Build history of the part. All positions in model axes, mm. A direction names the side the tool comes from. Coordinates: 2 decimals unless noted, no trailing zeros. Write each loop counter-clockwise with the first axis right and the second up, starting at its lowest first coordinate (ties: lowest second). Pieces come first, ordered by that corner, then holes.
```python
from build123d import *

# Parameters (mm, degrees)
SKETCH_1_R                  = 7.5
SKETCH_1_R_2                = 6
EXTRUDE_1_DEPTH             = 17
CUT_EXTRUDE_1_REACH         = 25.88
CUT_EXTRUDE_1_END_RADIUS    = 6
SKETCH_2_W                  = 1
SKETCH_2_H                  = 17
SKETCH_3_W                  = 4
SKETCH_3_H                  = 17
EXTRUDE_2_DEPTH             = 5
EXTRUDE_2_DIRECTION_2_REACH = 25.88
CUT_EXTRUDE_START           = -2
CUT_EXTRUDE_4_DEPTH         = 2
CUT_EXTRUDE_2_REACH         = 26.274
SKETCH_4_R                  = 1.25
CUT_EXTRUDE_3_DEPTH         = 1.5
EXTRUDE_6_DEPTH             = 5
SKETCH_13_W                 = 4.5
SKETCH_13_H                 = 12.5
EXTRUDE_7_DEPTH             = 5
CUT_EXTRUDE_5_REACH         = 34.2
SKETCH_11_R                 = 1.1
FILLET_1_R                  = 1.5


with BuildPart() as part:
    # 草图1 → 凸台-拉伸1 (new body)
    with BuildSketch(Plane(origin=(0, 0, 0), x_dir=(1, 0, 0), z_dir=(0, 1, 0))):
        with Locations(Location((0, 0, 0), (0, 0, 270))):
            Circle(SKETCH_1_R)
        with Locations(Location((0, 0, 0), (0, 0, 270))):
            Circle(SKETCH_1_R_2, mode=Mode.SUBTRACT)
    extrude(amount=EXTRUDE_1_DEPTH)

    # 切除-拉伸1: up to this cylinder (the profile starts outside it)
    cut_extrude_1_end = Plane(origin=(0, 8.5, 0), z_dir=(0, -1, 0)) * Cylinder(CUT_EXTRUDE_1_END_RADIUS, 64.76, mode=Mode.PRIVATE)
    # 草图2 → 切除-拉伸1 (cut, up to the surface)
    with BuildSketch(Plane.XY.offset(7.5), mode=Mode.PRIVATE) as cut_extrude_1_sk1:
        with Locations((0, 8.5)):
            Rectangle(SKETCH_2_W, SKETCH_2_H)
    cut_extrude_1_tool1 = extrude(cut_extrude_1_sk1.sketch, amount=-CUT_EXTRUDE_1_REACH, mode=Mode.PRIVATE) - cut_extrude_1_end
    add(cut_extrude_1_tool1.solids().sort_by_distance((0, 8.5, 7.5))[0], mode=Mode.SUBTRACT)

    # 草图3 → 凸台-拉伸2 (add)
    with BuildSketch(Plane.XY.offset(7.5)):
        with Locations((-2.5, 8.5)):
            Rectangle(SKETCH_3_W, SKETCH_3_H)
        with Locations((2.5, 8.5)):
            Rectangle(SKETCH_3_W, SKETCH_3_H)
    extrude(amount=EXTRUDE_2_DEPTH)

    # 草图3 → 凸台-拉伸2 direction 2 (add, up to next)
    with BuildSketch(Plane.XY.offset(7.5), mode=Mode.PRIVATE) as extrude_2_direction_2_sk1:
        with Locations((-2.5, 8.5)):
            Rectangle(SKETCH_3_W, SKETCH_3_H)
    extrude_2_direction_2_tool1 = extrude(extrude_2_direction_2_sk1.sketch, amount=-EXTRUDE_2_DIRECTION_2_REACH, mode=Mode.PRIVATE) - part.part
    # 草图3 → 凸台-拉伸2 direction 2 (add, up to next)
    with BuildSketch(Plane.XY.offset(7.5), mode=Mode.PRIVATE) as extrude_2_direction_2_sk2:
        with Locations((2.5, 8.5)):
            Rectangle(SKETCH_3_W, SKETCH_3_H)
    extrude_2_direction_2_tool2 = extrude(extrude_2_direction_2_sk2.sketch, amount=-EXTRUDE_2_DIRECTION_2_REACH, mode=Mode.PRIVATE) - part.part
    add(extrude_2_direction_2_tool1.solids().sort_by_distance((-2.5, 8.5, 7.5))[0])
    add(extrude_2_direction_2_tool2.solids().sort_by_distance((2.5, 8.5, 7.5))[0])

    # 草图7 → 切除-拉伸4 (cut)
    with BuildSketch(Plane(origin=(0, 17, 0), x_dir=(1, 0, 0), z_dir=(0, 1, 0)).offset(CUT_EXTRUDE_START)):
        with BuildLine():
            Line((-4.5, -6), (-4.5, -12.5))
            Line((-4.5, -12.5), (4.5, -12.5))
            Line((4.5, -12.5), (4.5, -6))
            ThreePointArc((4.5, -6), (0, -7.5), (-4.5, -6))
        make_face()
    extrude(amount=CUT_EXTRUDE_4_DEPTH, mode=Mode.SUBTRACT)

    # 切除-拉伸2: up to this face of the body (flat: up to its plane)
    cut_extrude_2_end = Plane(part.part.faces().sort_by_distance((4.5, 7.5, 9.25))[0])
    # 草图4 → 切除-拉伸2 (cut, up to the picked face)
    with BuildSketch(Plane.ZY.offset(4.5), mode=Mode.PRIVATE) as cut_extrude_2_sk1:
        with Locations(Location((9.25, 11.5, 0), (0, 0, 270))):
            Circle(SKETCH_4_R)
    cut_extrude_2_tool1 = split(extrude(cut_extrude_2_sk1.sketch, amount=-CUT_EXTRUDE_2_REACH, mode=Mode.PRIVATE), bisect_by=cut_extrude_2_end, keep=Keep.BOTH, mode=Mode.PRIVATE)
    # 草图4 → 切除-拉伸2 (cut, up to the picked face)
    with BuildSketch(Plane.ZY.offset(4.5), mode=Mode.PRIVATE) as cut_extrude_2_sk2:
        with Locations(Location((9.25, 3.5, 0), (0, 0, 270))):
            Circle(SKETCH_4_R)
    cut_extrude_2_tool2 = split(extrude(cut_extrude_2_sk2.sketch, amount=-CUT_EXTRUDE_2_REACH, mode=Mode.PRIVATE), bisect_by=cut_extrude_2_end, keep=Keep.BOTH, mode=Mode.PRIVATE)
    add(cut_extrude_2_tool1.solids().sort_by(Axis((-4.5, 11.5, 9.25), (1, 0, 0)))[0], mode=Mode.SUBTRACT)
    add(cut_extrude_2_tool2.solids().sort_by(Axis((-4.5, 3.5, 9.25), (1, 0, 0)))[0], mode=Mode.SUBTRACT)

    # 草图5 → 切除-拉伸3 (cut)
    with BuildSketch(Plane(origin=(4.5, 0, 0), x_dir=(0, 0, -1), z_dir=(1, 0, 0))):
        Polygon((-9.25, 9.190598923), (-7.25, 10.345299462), (-7.25, 12.654700538), (-9.25, 13.809401077), (-11.25, 12.654700538), (-11.25, 10.345299462), align=None)
        Polygon((-9.25, 1.190598923), (-7.25, 2.345299462), (-7.25, 4.654700538), (-9.25, 5.809401077), (-11.25, 4.654700538), (-11.25, 2.345299462), align=None)
    extrude(amount=-CUT_EXTRUDE_3_DEPTH, mode=Mode.SUBTRACT)

    # 草图12 → 凸台-拉伸6 (add)
    with BuildSketch(Plane(origin=(0, 0, 0), x_dir=(1, 0, 0), z_dir=(0, 1, 0))):
        Polygon((-10.8, 7.5), (22.2, 7.5), (22.2, 2.5), (7.071067812, 2.5), (0, 7.208487923), (-7.071067812, 2.5), (-10.8, 2.5), align=None)
    extrude(amount=EXTRUDE_6_DEPTH)

    # 草图13 → 凸台-拉伸7 (add)
    with BuildSketch(Plane(origin=(0, 0, 0), x_dir=(1, 0, 0), z_dir=(0, 1, 0))):
        with Locations((-8.55, 13.75)):
            Rectangle(SKETCH_13_W, SKETCH_13_H)
        with Locations((19.95, 13.75)):
            Rectangle(SKETCH_13_W, SKETCH_13_H)
    extrude(amount=EXTRUDE_7_DEPTH)

    # 草图11 → 切除-拉伸5 (cut, up to next)
    with BuildSketch(Plane(origin=(0, 5, 0), x_dir=(1, 0, 0), z_dir=(0, 1, 0)), mode=Mode.PRIVATE) as cut_extrude_5_sk1:
        with Locations(Location((-8.55, 13.75, 0), (0, 0, 270))):
            Circle(SKETCH_11_R)
    cut_extrude_5_tool1 = extrude(cut_extrude_5_sk1.sketch, amount=-CUT_EXTRUDE_5_REACH, mode=Mode.PRIVATE) & part.part
    # 草图11 → 切除-拉伸5 (cut, up to next)
    with BuildSketch(Plane(origin=(0, 5, 0), x_dir=(1, 0, 0), z_dir=(0, 1, 0)), mode=Mode.PRIVATE) as cut_extrude_5_sk2:
        with Locations(Location((19.95, 13.75, 0), (0, 0, 270))):
            Circle(SKETCH_11_R)
    cut_extrude_5_tool2 = extrude(cut_extrude_5_sk2.sketch, amount=-CUT_EXTRUDE_5_REACH, mode=Mode.PRIVATE) & part.part
    add(cut_extrude_5_tool1.solids().sort_by_distance((-8.55, 5, -13.75))[0], mode=Mode.SUBTRACT)
    add(cut_extrude_5_tool2.solids().sort_by_distance((19.95, 5, -13.75))[0], mode=Mode.SUBTRACT)

    # 圆角1
    fillet_1_edges = [part.edges().sort_by_distance(p)[0] for p in [
        (-10.8, 2.5, -2.5),
        (-7.071067812, 2.5, -2.5),
        (7.071067812, 2.5, -2.5),
        (22.2, 2.5, -2.5),
        (-10.8, 2.5, -20),
        (-6.3, 2.5, -20),
        (22.2, 2.5, -20),
        (17.7, 2.5, -20),
    ]]
    fillet(fillet_1_edges, radius=FILLET_1_R)


solid = part.part
```
1. Flat gauge pins, fed straight in: pin 1 (1.5 mm diameter, centred on y = 3.5, z = 9.25, fed in from -X); pin 2 (3 mm diameter, centred on x = -3, z = 10, fed in from +Y); pin 3 (2 mm diameter, centred on x = 9.5, y = 4.5, fed in from -Z); pin 4 (10 mm diameter, centred on y = 12.5, z = -4, fed in from +X). Where does each tip first touch, or does it go through?
Computed values:
pin 1: passes through
pin 2: stops at y = 15
pin 3: stops at z = -7.5
pin 4: stops at x = 7.5
2. Mould opens along X. For faces 5 (the face through (2, 8, 12.5)), 6 (the face through (-7.838, 2.535, -2.013)), 7 (the face through (0, 8, -6)), 8 (the face through (-0.5, 8, 9)) say: +X half, -X half, draft (parallel to the pull), parting line (faces both ways), or undercut.
Computed values:
face 5: draft
face 6: -X half
face 7: undercut
face 8: undercut
3. Probe line 1 along X through (y, z) = (14.75, 11.5); line 2 along X through (y, z) = (12.75, 11); line 3 along Z through (x, y) = (-1.5, 3.5). List the from-to ranges inside material, lowest first.
Computed values:
line 1: x = -4.5 to -0.5, 0.5 to 4.5
line 2: x = -4.5 to -0.5, 0.5 to 3
line 3: z = -7.5 to -5.81, 5.81 to 8, 10.5 to 12.5
4. Saw through at B-B on x = 1.5. List the corners of the cut face in (y, z).
Computed values:
outline: (0, -7.5) - (5, -7.5) - (5, -7.35) - (17, -7.35) - (17, -5.81) - (0, -5.81) - close; (0, 5.81) - (17, 5.81) - (17, 7.35) - (15, 7.35) - (15, 12.5) - (0, 12.5) - close; hole circle Ø2.5 at (3.5, 9.25); hole circle Ø2.5 at (11.5, 9.25)
5. Saw through at A-A on z = 0. List the corners of the cut face in (x, y).
Computed values:
outline: (-7.5, 0) - (-6, 0) - (-6, 17) - (-7.5, 17) - close; (6, 0) - (7.5, 0) - (7.5, 17) - (6, 17) - close
6. Saw through at D-D on x = 19.95. List the corners of the cut face in (y, z), plus the area to 3 significant figures.
Computed values:
outline: (0, -20) - (5, -20) - (5, -14.85) - (0, -14.85) - close; (0, -12.65) - (5, -12.65) - (5, -2.5) - (0, -2.5) - close
area: 76.5 mm2
7. Saw through at C-C on y = 11.5. List the corners of the cut face in (x, z).
Computed values:
outline: (-4.5, 6) arc R7.5 ccw (long way) to (4.5, 6) - (4.5, 7.25) - (3, 7.25) - (3, 8) - (0.5, 8) - (0.5, 5.98) arc R6 cw (long way) to (-0.5, 5.98) - (-0.5, 8) - (-4.5, 8) - close; (-4.5, 10.5) - (-0.5, 10.5) - (-0.5, 12.5) - (-4.5, 12.5) - close; (0.5, 10.5) - (3, 10.5) - (3, 11.25) - (4.5, 11.25) - (4.5, 12.5) - (0.5, 12.5) - close
8. 3-axis set-ups, long thin cutter, end or side, ignore diameter. For faces 1 (the face through (4.5, 7, 9)), 2 (the face through (4, 0, -6)), 3 (the face through (4, 4, 11.25)), 4 (the face through (-6.75, 2.54, -19.57)): which of +Z, -Z, +X, -X, +Y, -Y reach the whole face in a straight line?
Computed values:
face 1: +Z, +X, +Y, -Y
face 2: +Z, -Z, +X, -X, -Y
face 3: +X
face 4: -Z, +Y, -Y
